The figure shows three views and two pictorial views of one solid part (mm, origin at its lowest corner). Answer the questions. A direction names the side the tool comes from. Coordinates: 2 decimals unless noted, no trailing zeros. Write each loop counter-clockwise with the first axis right and the second up, starting at its lowest first coordinate (ties: lowest second). Pieces come first, ordered by that corner, then holes. Notation, with made-up numbers: (6, -2.75) - (28, -2.75) arc R19 cw to (28, 29.25) - close; hole circle Ø3 at (72, 14.25). An arc over 180 degrees is marked (long way). Use a Markdown table: item, result. Add a question column.
(1) For a pull along Z with two mould halves and no side action, classify the marked faces 3, 4 and 5 as released by +Z, released by -Z, zero draft, split by the parting line, or undercut.
(2) Find the intervals of material crossed by line 1 (Y direction, x = 8, z = 12.25); line 2 (Z direction, x = 2, y = 6.5), in increasing order. Write a range as from..to.
(3) A tool of negligible diameter and unlimited length cuts with its end or side. For the marked faces 1 and 2, from which of +Z, -Z, +X, -X, +Y, -Y can it reach the whole face along a straight path? Write none if from no direction.
(4) The part is cut by section C-C, the plane z = 6.5. Give the vertices of the cut face in (x, y).
(5) The part is cut by section A-A, the plane x = 8. Give the vertices of the cut face in (y, z).
(6) Given pin 1 Ø3 at (x, y) = (8, 8) entering from -Z; pin 2 Ø1.5 at (x, z) = (3.5, 13.5) entering from -Y; pin 3 Ø2 at (y, z) = (7.5, 12) entering from +X; pin 4 Ø2 at (x, z) = (9.5, 7.5) entering from -Y, each flat-ended and moving along its own axis, determine where each tip first touches the part or whether it passes through.
(7) The part is cut by section D-D, the plane x = 12.25. Give the vertices of the cut face in (y, z).
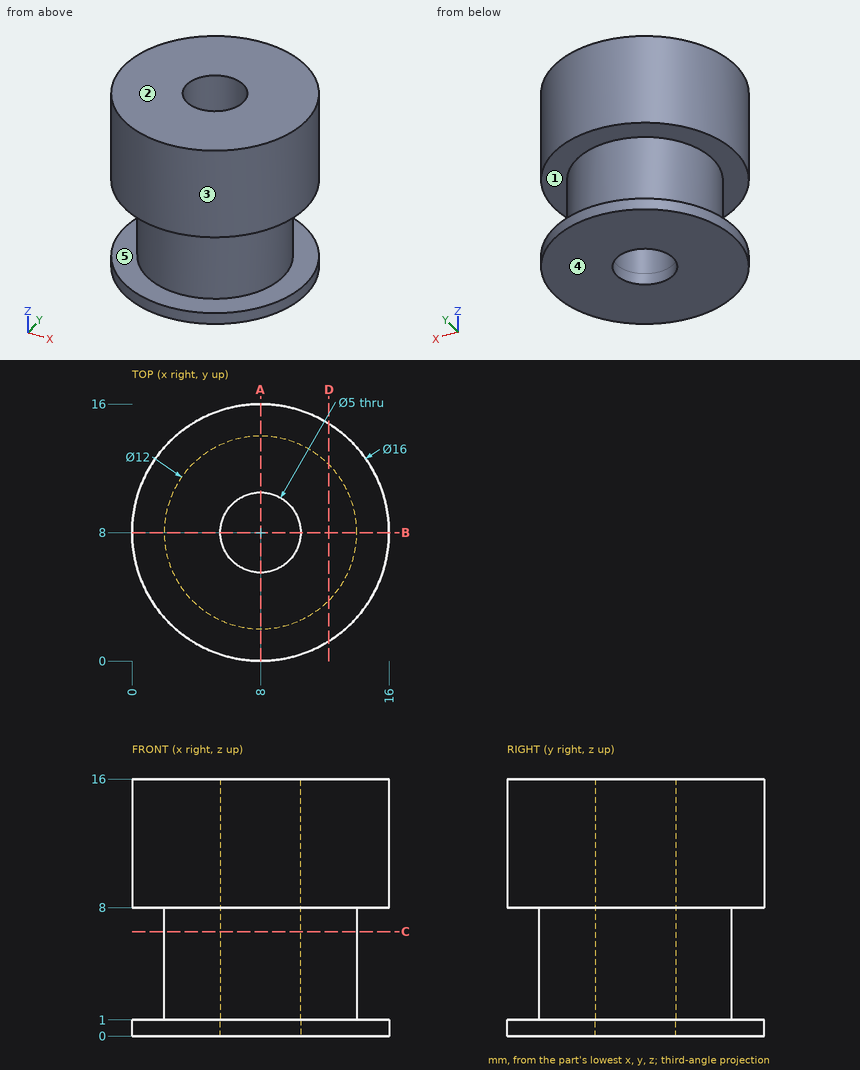
Model answer:
| question | item | result |
|---|---|---|
| 1 | face 3 | zero draft |
| 1 | face 4 | released by -Z |
| 1 | face 5 | undercut |
| 2 | line 1 | 0..5.5, 10.5..16 |
| 2 | line 2 | 0..1, 8..16 |
| 3 | face 1 | none |
| 3 | face 2 | +Z, +X, -X, +Y, -Y |
| 4 | outline | circle Ø12 at (8, 8); hole circle Ø5 at (8, 8) |
| 5 | outline | (0, 0) - (5.5, 0) - (5.5, 16) - (0, 16) - (0, 8) - (2, 8) - (2, 1) - (0, 1) - close; (10.5, 0) - (16, 0) - (16, 1) - (14, 1) - (14, 8) - (16, 8) - (16, 16) - (10.5, 16) - close |
| 6 | pin 1 | through |
| 6 | pin 2 | y = 0.93 |
| 6 | pin 3 | x = 16 |
| 6 | pin 4 | y = 0.03 |
| 7 | outline | (1.22, 0) - (14.78, 0) - (14.78, 1) - (12.24, 1) - (12.24, 8) - (14.78, 8) - (14.78, 16) - (1.22, 16) - (1.22, 8) - (3.76, 8) - (3.76, 1) - (1.22, 1) - close |
